from build123d import *

# Parameters (mm, degrees)
F0_W      = 15
F0_H      = 55
F1_DEPTH  = 5
F2_W      = 10
F2_H      = 30
F3_DEPTH  = 25
F4_R      = 11
F5_DEPTH  = 7
F6_R      = 2
F6_R_2    = 2.05
F7_DEPTH  = 25
F8_R      = 2
F9_R      = 7
F10_DEPTH = 5.501


with BuildPart() as f1:
    # F0 (on Top) → F1 (new body)
    with BuildSketch(Plane.XY):
        Rectangle(F0_W, F0_H)
    extrude(amount=F1_DEPTH)

    # F2 (on face) → F3 (join)
    with BuildSketch(Plane.XY.offset(5)):
        Rectangle(F2_W, F2_H)
    extrude(amount=F3_DEPTH)

    # F4 (on face) → F5 (cut)
    with BuildSketch(Plane.YZ.offset(5)):
        with Locations((0, 17.5)):
            Circle(F4_R)
    extrude(amount=-F5_DEPTH, mode=Mode.SUBTRACT)

    # F6 (on face) → F7 (cut)
    with BuildSketch(Plane.XY.offset(5)):
        with Locations((0, -23.5)):
            Circle(F6_R)
        with Locations((0, 23.5)):
            Circle(F6_R_2)
    extrude(amount=-F7_DEPTH, mode=Mode.SUBTRACT)

    # F8
    f8_edges = [f1.edges().sort_by_distance(p)[0] for p in [
        (0, -15, 30),
        (0, -15, 5),
        (5, 0, 5),
        (0, 15, 30),
        (0, 15, 5),
        (-5, 0, 5),
    ]]
    fillet(f8_edges, radius=F8_R)

    # F9 (on face) → F10 (cut, through all)
    with BuildSketch(Plane.YZ.offset(-2)):
        with Locations((0, 17.5)):
            Circle(F9_R)
    extrude(amount=-F10_DEPTH, mode=Mode.SUBTRACT)


solid = f1.part
Geometry check sheet. Reference: the model listing, model coordinates, mm. A direction names the side the tool comes from. Coordinates: 2 decimals unless noted, no trailing zeros. Loops run counter-clockwise (first coordinate to the right, second up) from the corner with the lowest first, then second, coordinate; pieces in that order, holes last. Notation, with made-up numbers: (-24, 63) - (-17, 63) arc R19 ccw to (-17, 67) - close; hole circle Ø8 at (31.25, 46). An arc over 180 degrees is marked (long way). Use one line per item in the form item = value. Start each with the question number.
Item 1: Section check D-D, the plane z = 15.75. Enter the section's corners in (x, y).
Item 2: Tool access check on faces 4 (the face through (0, 15, 17)), 5 (the face through (-2, 7.2, 17.7)), 6 (the face through (5, 0, 29)), 7 (the face through (-5, -7, 21)). Record the directions out of +Z, -Z, +X, -X, +Y, -Y that give a thin tool (end or side, any length) a straight path to the whole face; none if there is none.
Item 3: Section check C-C, the plane x = -3.5. Enter the section's corners in (y, z).
Item 4: Section check B-B, the plane y = 23.5. Enter the section's corners in (x, z).
Item 5: Section check A-A, the plane x = 0. Enter the section's corners in (y, z), and give its area (3 significant figures).
Item 6: Gauge pin test, flat ends, axial feed: pin 1 (7 mm diameter, centred on y = 6.5, z = 23.5, fed in from +X); pin 2 (4 mm diameter, centred on x = -3, y = 18.5, fed in from +Z); pin 3 (3 mm diameter, centred on y = 2, z = 21.5, fed in from -X); pin 4 (6 mm diameter, centred on x = 0.5, y = -20, fed in from -Z). Record the tip position at first contact, or that the pin passes through.
Item 7: Mould release check, pull along X, two halves, no side actions. Record for faces 1 (the face through (-0.26, -21.517, 2.535)), 2 (the face through (5.6, 10.24, 5.57)), 3 (the face through (0, -15, 17)): +X half, -X half, draft (parallel to the pull), parting line (faces both ways), or undercut.
Item 8: Thickness scan on probe 1 along Y at (x, z) = (0, 3.85); probe 2 along Y at (x, z) = (2.5, 17.5); probe 3 along X at (y, z) = (13.5, 22.5). Record the ranges inside material, lowest first.
Computed:
q1.outline = (-5, -15) - (5, -15) - (5, -10.86) - (-2, -10.86) - (-2, -6.78) - (-5, -6.78) - close; (-5, 6.78) - (-2, 6.78) - (-2, 10.86) - (5, 10.86) - (5, 15) - (-5, 15) - close
q2.face_4 = +Z, +X, -X, +Y
q2.face_5 = +X
q2.face_6 = +Z, +X, +Y, -Y
q2.face_7 = +Z, -X, +Y, -Y
q3.outline = (-27.5, 0) - (27.5, 0) - (27.5, 5) - (17, 5) arc R2 cw to (15, 7) - (15, 28) arc R2 ccw to (13, 30) - (-13, 30) arc R2 ccw to (-15, 28) - (-15, 7) arc R2 cw to (-17, 5) - (-27.5, 5) - close; hole circle Ø14 at (0, 17.5)
q4.outline = (-7.5, 0) - (-2.05, 0) - (-2.05, 5) - (-7.5, 5) - close; (2.05, 0) - (7.5, 0) - (7.5, 5) - (2.05, 5) - close
q5.outline = (-27.5, 0) - (-25.5, 0) - (-25.5, 5) - (-27.5, 5) - close; (-21.5, 0) - (21.45, 0) - (21.45, 5) - (17, 5) arc R2 cw to (15, 7) - (15, 28) arc R2 ccw to (13, 30) - (-13, 30) arc R2 ccw to (-15, 28) - (-15, 7) arc R2 cw to (-17, 5) - (-21.5, 5) - close; (25.55, 0) - (27.5, 0) - (27.5, 5) - (25.55, 5) - close; hole circle Ø22 at (0, 17.5)
q5.area = 604 mm2
q6.pin_1 = 5
q6.pin_2 = 5.06
q6.pin_3 = through
q6.pin_4 = 0
q7.face_1 = undercut
q7.face_2 = +X half
q7.face_3 = draft
q8.probe_1 = -27.5 to -25.5, -21.5 to 21.45, 25.55 to 27.5
q8.probe_2 = -15 to -11, 11 to 15
q8.probe_3 = -5 to 5
